Check sheet for the modelled part. Datum: model origin and axes. Units: mm. Face numbers are marked on the shaded views. A direction names the side the tool comes from. Coordinates: 2 decimals unless noted, no trailing zeros. Write each loop counter-clockwise with the first axis right and the second up, starting at its lowest first coordinate (ties: lowest second). Pieces come first, ordered by that corner, then holes. Notation, with made-up numbers: M 73,-13.75 L 96,-13.75 A30 cw 96,16.25 Z; hole C 50,88 d9. An arc over 180 degrees is marked long. Answer as CSV lines item,"result". Start each with the question number.
1) Access from +Z, -Z, +X, -X, +Y, -Y to the whole of each face (thin tool, end or side, straight path). Record for the marked faces 1 and 2.
2) Section check A-A (x = -62.23). Record the cut outline in (y, z).
3) Material ranges on L1, parallel to Y at x = -62, z = 5; L2, parallel to X at y = 32.5, z = 5.5, recorded low to high. Write a range as [from, to].
4) Section check C-C (x = 0). Record the cut outline in (y, z).
5) Draft check along X on the marked faces 3, 4 and 5. Enter one of: +X half, -X half, draft (parallel to the pull), parting line (faces both ways), or undercut.
6) Section check B-B (y = 0). Record the cut outline in (x, z).
7) Go/stop test with flat-tipped pins: pin 1 Ø4 at (x, y) = (57, -12.5) entering from +Z; pin 2 Ø12 at (y, z) = (17, 60.5) entering from +X; pin 3 Ø3 at (y, z) = (-11, 42.5) entering from -X. Record where each tip stops, or that it passes through.
8) Section check D-D (z = 12). Record the cut outline in (x, y).
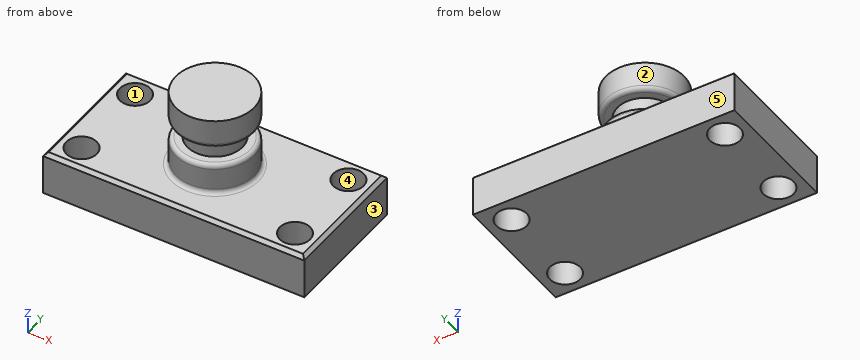
from build123d import *

# Parameters (mm, degrees)
F0_W     = 152.4
F0_H     = 76.2
F1_DEPTH = 25.4
F2_R     = 8.89
F3_DEPTH = 25.4
F4_SIZE  = 2.032
F5_W     = 22.86
F5_H     = 45.72
F7_W     = 6.9182990119
F7_H     = 11.1455507576
F9_R     = 2.54
F10_R    = 2.54


with BuildPart() as f1:
    # F0 (on Top) → F1 (new body)
    with BuildSketch(Plane.XY):
        Rectangle(F0_W, F0_H)
    extrude(amount=F1_DEPTH)

    # F2 (on face) → F3 (cut)
    with BuildSketch(Plane.XY.offset(25.4)):
        with Locations((-62.23, 24.638)):
            Circle(F2_R)
        with Locations((62.23, -24.638)):
            Circle(F2_R)
        with Locations((62.23, 24.638)):
            Circle(F2_R)
        with Locations((-62.23, -24.638)):
            Circle(F2_R)
    extrude(amount=-F3_DEPTH, mode=Mode.SUBTRACT)

    # F4
    f4_edges = [f1.edges().sort_by_distance(p)[0] for p in [
        (76.2, 0, 25.4),
        (0, 38.1, 25.4),
        (0, -38.1, 25.4),
        (-76.2, 0, 25.4),
    ]]
    chamfer(f4_edges, length=F4_SIZE)

    # F5 (on Front) → F6 (revolve)
    with BuildSketch(Plane.XZ):
        with Locations((11.43, 48.26)):
            Rectangle(F5_W, F5_H)
    revolve(axis=Axis((0, 0, 48.26), (0, 0, 1)))

    # F7 (on Front) → F8 (revolve, cut)
    with BuildSketch(Plane.XZ):
        with Locations((19.5512440987, 48.6171673983)):
            Rectangle(F7_W, F7_H)
    revolve(axis=Axis((0, 0, 25.4), (0, 0, 1)), mode=Mode.SUBTRACT)

    # F9
    f9_edges = [f1.edges().sort_by_distance(p)[0] for p in [
        (22.86, 0, 34.222196),
        (-22.86, 0, 43.044392),
        (-22.86, 0, 25.4),
    ]]
    fillet(f9_edges, radius=F9_R)

    # F10
    f10_edges = [f1.edges().sort_by_distance(p)[0] for p in [
        (-22.86, 0, 54.189943),
    ]]
    fillet(f10_edges, radius=F10_R)


solid = f1.part
Results found:
1,face 1,"+Z, -Z"
1,face 2,"+Z"
2,outline,"M -38.1,0 L -33.53,0 L -33.53,25.4 L -36.07,25.4 L -38.1,23.37 Z; M -15.75,0 L 15.75,0 L 15.75,25.4 L -15.75,25.4 Z; M 33.53,0 L 38.1,0 L 38.1,23.37 L 36.07,25.4 L 33.53,25.4 Z"
3,L1,"y = [-38.1, -33.53], [-15.75, 15.75], [33.53, 38.1]"
3,L2,"x = [-76.2, -66.38], [-58.08, 58.08], [66.38, 76.2]"
4,outline,"M -38.1,0 L 38.1,0 L 38.1,23.37 L 36.07,25.4 L 25.4,25.4 A2.54 cw 22.86,27.94 L 22.86,40.5 A2.54 ccw 20.32,43.04 L 16.09,43.04 L 16.09,54.19 L 20.32,54.19 A2.54 ccw 22.86,56.73 L 22.86,71.12 L -22.86,71.12 L -22.86,56.73 A2.54 ccw -20.32,54.19 L -16.09,54.19 L -16.09,43.04 L -20.32,43.04 A2.54 ccw -22.86,40.5 L -22.86,27.94 A2.54 cw -25.4,25.4 L -36.07,25.4 L -38.1,23.37 Z"
5,face 3,"+X half"
5,face 4,"undercut"
5,face 5,"draft"
6,outline,"M -76.2,0 L 76.2,0 L 76.2,23.37 L 74.17,25.4 L 25.4,25.4 A2.54 cw 22.86,27.94 L 22.86,40.5 A2.54 ccw 20.32,43.04 L 16.09,43.04 L 16.09,54.19 L 20.32,54.19 A2.54 ccw 22.86,56.73 L 22.86,71.12 L -22.86,71.12 L -22.86,56.73 A2.54 ccw -20.32,54.19 L -16.09,54.19 L -16.09,43.04 L -20.32,43.04 A2.54 ccw -22.86,40.5 L -22.86,27.94 A2.54 cw -25.4,25.4 L -74.17,25.4 L -76.2,23.37 Z"
7,pin 1,"stops at z = 25.4"
7,pin 2,"stops at x = 20.04"
7,pin 3,"stops at x = -20.39"
8,outline,"M -76.2,-38.1 L 76.2,-38.1 L 76.2,38.1 L -76.2,38.1 Z; hole C -62.23,-24.64 d17.78; hole C -62.23,24.64 d17.78; hole C 62.23,-24.64 d17.78; hole C 62.23,24.64 d17.78"
